```python
from build123d import *

# Parameters (mm, degrees)
SKETCH1_W                   = 12.7
SKETCH1_H                   = 38.1
BOSS_EXTRUDE1_DEPTH         = 19.05
FILLET2_RADIUS              = 6.35
FILLET2_LENGTH              = 38.1
SKETCH2_R                   = 3.81
CUT_EXTRUDE1_DEPTH          = 38.1
CUT_EXTRUDE2_DEPTH          = 6.35
MIRROR7_COPY_1_DEPTH        = 6.35
FILLET2_OF_MIRROR7_2_RADIUS = 6.35
FILLET2_OF_MIRROR7_2_LENGTH = 38.1


with BuildPart() as part:
    # Sketch1 → Boss-Extrude1 (new, symmetric)
    with BuildSketch(Plane.XY):
        Rectangle(SKETCH1_W, SKETCH1_H)
    boss_extrude1 = extrude(amount=BOSS_EXTRUDE1_DEPTH, both=True)

    # Fillet2: full round fillet: the end face becomes a half cylinder, R = half its width
    fillet2_face = Plane((0, -19.05, 0), x_dir=(0, 0, 1), z_dir=(0, -1, 0))  # on the end face: x along it, z out of the body
    fillet2_slab = fillet2_face.offset(-FILLET2_RADIUS / 2) * Box(FILLET2_LENGTH, 2 * FILLET2_RADIUS, FILLET2_RADIUS, mode=Mode.PRIVATE)  # the body's end, R deep
    fillet2_round = Plane((0, -12.7, 0), x_dir=(0, -1, 0), z_dir=(0, 0, 1)) * Cylinder(FILLET2_RADIUS, FILLET2_LENGTH, mode=Mode.PRIVATE)  # its axis R under the face
    add(fillet2_slab - fillet2_round, mode=Mode.SUBTRACT)

    # Sketch2 → Cut-Extrude1 (cut)
    with BuildSketch(Plane.XY.offset(19.05)):
        with Locations((0, -12.7)):
            Circle(SKETCH2_R)
    cut_extrude1 = extrude(amount=-CUT_EXTRUDE1_DEPTH, mode=Mode.SUBTRACT)

    # Sketch8 → Cut-Extrude2 (cut)
    with BuildSketch(Plane.XY.offset(19.05)):
        with BuildLine():
            Line((-12.7, 19.05), (-12.7, -58.61254398))
            Line((-12.7, -58.61254398), (12.7, -58.61254398))
            Line((12.7, -58.61254398), (12.7, 19.05))
            ThreePointArc((12.7, 19.05), (0, 6.35), (-12.7, 19.05))
        make_face()
    cut_extrude2 = extrude(amount=-CUT_EXTRUDE2_DEPTH, mode=Mode.SUBTRACT)

    # Mirror5: Cut-Extrude2 across plane
    add(cut_extrude2.mirror(Plane.XY), mode=Mode.SUBTRACT)

    # Mirror7: Boss-Extrude1, Cut-Extrude1, Cut-Extrude2 across plane
    add(boss_extrude1.mirror(Plane(origin=(-6.35, 19.05, 19.05), x_dir=(0, 0, 1), z_dir=(0, -1, 0))))
    add(cut_extrude1.mirror(Plane(origin=(-6.35, 19.05, 19.05), x_dir=(0, 0, 1), z_dir=(0, -1, 0))), mode=Mode.SUBTRACT)
    add(cut_extrude2.mirror(Plane(origin=(-6.35, 19.05, 19.05), x_dir=(0, 0, 1), z_dir=(0, -1, 0))), mode=Mode.SUBTRACT)

    # Mirror7 copy 1 sketch → Mirror7 copy 1 (cut)
    with BuildSketch(Plane(origin=(0, 38.1, -19.05), x_dir=(1, 0, 0), z_dir=(0, 0, -1))):
        with BuildLine():
            Line((-12.7, 19.05), (-12.7, -58.61254398))
            Line((-12.7, -58.61254398), (12.7, -58.61254398))
            Line((12.7, -58.61254398), (12.7, 19.05))
            ThreePointArc((12.7, 19.05), (0, 6.35), (-12.7, 19.05))
        make_face()
    extrude(amount=-MIRROR7_COPY_1_DEPTH, mode=Mode.SUBTRACT)

    # Fillet2 of Mirror7 2: full round fillet: the end face becomes a half cylinder, R = half its width
    fillet2_of_mirror7_2_face = Plane((0, 57.15, 0), x_dir=(0, 0, 1), z_dir=(0, 1, 0))  # on the end face: x along it, z out of the body
    fillet2_of_mirror7_2_slab = fillet2_of_mirror7_2_face.offset(-FILLET2_OF_MIRROR7_2_RADIUS / 2) * Box(FILLET2_OF_MIRROR7_2_LENGTH, 2 * FILLET2_OF_MIRROR7_2_RADIUS, FILLET2_OF_MIRROR7_2_RADIUS, mode=Mode.PRIVATE)  # the body's end, R deep
    fillet2_of_mirror7_2_round = Plane((0, 50.8, 0), x_dir=(0, 1, 0), z_dir=(0, 0, 1)) * Cylinder(FILLET2_OF_MIRROR7_2_RADIUS, FILLET2_OF_MIRROR7_2_LENGTH, mode=Mode.PRIVATE)  # its axis R under the face
    add(fillet2_of_mirror7_2_slab - fillet2_of_mirror7_2_round, mode=Mode.SUBTRACT)


solid = part.part
```
Work out the finished part from the listing and answer in its coordinate system (mm). A direction names the side the tool comes from. Coordinates: 2 decimals unless noted, no trailing zeros. Write each loop counter-clockwise with the first axis right and the second up, starting at its lowest first coordinate (ties: lowest second). Pieces come first, ordered by that corner, then holes.
Q1. Determine the mould class of faces 5 (the face through (-0.496, 47.022, 0.178)), 6 (the face through (6.35, 19, 0)), 7 (the face through (-0.14, -19.05, 0.18)) for opening direction Y: released by +Y, released by -Y, zero draft, split by the parting line, or undercut.
Q2. A cutting plane is placed at C-C, the plane y = -4. Give the vertices of the cut face in (x, z), then the cut area to 3 significant figures.
Q3. Find the intervals of material crossed by line 1 (Y direction, x = 0, z = 5); line 2 (Y direction, x = -1.5, z = 9); line 3 (Z direction, x = -4, y = 40.5), in increasing order.
Q4. A cutting plane is placed at D-D, the plane z = -15.5. Give the vertices of the cut face in (x, y), then the cut area to 3 significant figures.
Q5. A cutting plane is placed at B-B, the plane z = -6. Give the vertices of the cut face in (x, y), then the cut area to 3 significant figures.
Q6. A cutting plane is placed at A-A, the plane x = 0. Give the vertices of the cut face in (y, z).
Q7. Each of these flat-tipped pins is pushed along its axis until it touches: pin 1 Ø4 at (x, y) = (1.5, 38) entering from +Z; pin 2 Ø4 at (x, y) = (-3, -7) entering from -Z; pin 3 Ø1 at (x, z) = (-4, -7) entering from -Y. Where does it stop, or does it pass through?
Q8. Which of the six approach directions +Z, -Z, +X, -X, +Y, -Y give full straight-line access (tool end or side, diameter ignored) to faces 1 (the face through (0.09, 31.75, 15.92)), 2 (the face through (0.09, 31.75, -15.92)), 3 (the face through (0.09, 6.35, 15.92)), 4 (the face through (0.09, 6.35, -15.92))?
Findings below:
1. face 5: undercut
1. face 6: zero draft
1. face 7: released by -Y
2. outline: (-6.35, -12.7) - (6.35, -12.7) - (6.35, 12.7) - (-6.35, 12.7) - close
2. area: 323 mm2
3. line 1: y = -19.05 to -16.51, -8.89 to 46.99, 54.61 to 57.15
3. line 2: y = -18.87 to -16.2, -9.2 to 47.3, 54.3 to 56.97
3. line 3: z = -12.7 to 12.7
4. outline: (-6.35, 8.05) arc R12.7 ccw to (6.35, 8.05) - (6.35, 30.05) arc R12.7 ccw to (-6.35, 30.05) - close
4. area: 309 mm2
5. outline: (-6.35, -12.7) arc R6.35 ccw to (6.35, -12.7) - (6.35, 50.8) arc R6.35 ccw to (-6.35, 50.8) - close; hole circle Ø7.62 at (0, -12.7); hole circle Ø7.62 at (0, 50.8)
5. area: 842 mm2
6. outline: (-19.05, -12.7) - (-16.51, -12.7) - (-16.51, 12.7) - (-19.05, 12.7) - close; (-8.89, -12.7) - (6.35, -12.7) - (6.35, -19.05) - (31.75, -19.05) - (31.75, -12.7) - (46.99, -12.7) - (46.99, 12.7) - (31.75, 12.7) - (31.75, 19.05) - (6.35, 19.05) - (6.35, 12.7) - (-8.89, 12.7) - close; (54.61, -12.7) - (57.15, -12.7) - (57.15, 12.7) - (54.61, 12.7) - close
7. pin 1: stops at z = 12.7
7. pin 2: stops at z = -12.7
7. pin 3: stops at y = -18
8. face 1: +Z, +Y
8. face 2: -Z, +Y
8. face 3: +Z, -Y
8. face 4: -Z, -Y
